Geometry: final body of the model. Coordinates: model frame, mm. Face numbers are marked on the shaded views. A direction names the side the tool comes from. Give positions to 0.01 mm unless a question says otherwise; leave off trailing zeros. Order: outer loops, then holes, each group sorted by start corner. A loop starts at its lowest first (then second) coordinate and runs counter-clockwise, first axis right, second up. Notation, with made-up numbers: M 88,63 L 123,63 A10 cw 123,69 Z; hole C 30.25,10 d11. An arc over 180 degrees is marked long. Write item = value, one per line. Start each with the question number.
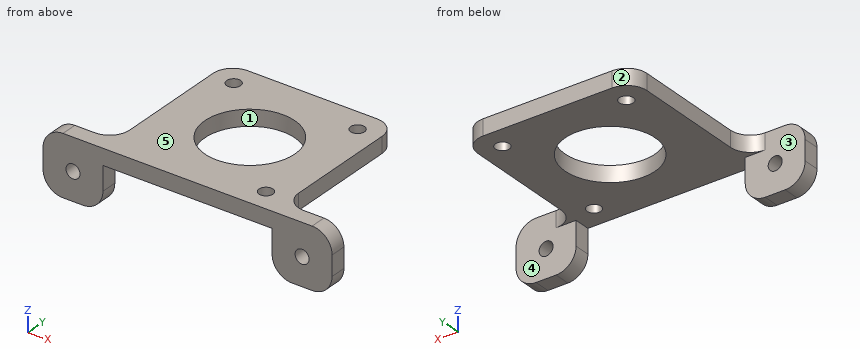
from build123d import *

# Parameters (mm, degrees)
F0_W     = 42.3
F0_H     = 42.2228726387
F0_R     = 1.75
F0_R_2   = 11.25
F1_DEPTH = 4
F2_W     = 15
F2_H     = 4
F3_DEPTH = 15
F4_R     = 5
F5_R     = 1.75
F6_DEPTH = 4


with BuildPart() as f1:
    # F0 (on Top) → F1 (new body)
    with BuildSketch(Plane.XY):
        with Locations((0, 0.0385636806)):
            Rectangle(F0_W, F0_H)
        with Locations((15.495, -15.495)):
            Circle(F0_R, mode=Mode.SUBTRACT)
        Circle(F0_R_2, mode=Mode.SUBTRACT)
        with Locations((-15.495, 15.495)):
            Circle(F0_R, mode=Mode.SUBTRACT)
        with Locations((15.495, 15.495)):
            Circle(F0_R, mode=Mode.SUBTRACT)
    extrude(amount=F1_DEPTH)

    # F2 (on face) → F3 (join)
    with BuildSketch(Plane.XY.offset(4)):
        with Locations((-28.65, -19.0728726387)):
            Rectangle(F2_W, F2_H)
        with Locations((28.65, -19.0728726387)):
            Rectangle(F2_W, F2_H)
    extrude(amount=-F3_DEPTH)

    # F4
    f4_edges = [f1.edges().sort_by_distance(p)[0] for p in [
        (21.15, 21.15, 2),
        (-21.15, 21.15, 2),
        (-21.15, -17.072873, 2),
        (21.15, -17.072873, 2),
        (36.15, -19.072873, 4),
        (-36.15, -19.072873, 4),
        (36.15, -19.072873, -11),
        (21.15, -19.072873, -11),
        (-21.15, -19.072873, -11),
        (-36.15, -19.072873, -11),
    ]]
    fillet(f4_edges, radius=F4_R)

    # F5 (on face) → F6 (cut, through all)
    with BuildSketch(Plane.XZ.offset(21.0728726387)):
        with Locations((-28.65, -4)):
            Circle(F5_R)
        with Locations((28.65, -4)):
            Circle(F5_R)
    extrude(amount=-F6_DEPTH, mode=Mode.SUBTRACT)


solid = f1.part
1) Ray query, L1, parallel to Z at x = 28.65, y = -17.95; L2, parallel to Y at x = -28, z = 1.75; L3, parallel to X at y = 12.5, z = 1.25. Return the intervals inside material, ascending.
2) Draft query along X for the marked faces 1, 2 and 3. Return one class per face: pulls with the +X half, pulls with the -X half, needs draft (parallel to the pull), parting line crosses it, or undercut.
3) Cut plane A-A (y = 0). Return loops of the section in (x, z).
4) Access query for the marked faces 4 and 5. Directions: +Z, -Z, +X, -X, +Y, -Y. A direction counts if a zero-diameter tool reaches every point of the face in a straight line with its end or side. Return the directions, or none.
5) Cut plane D-D (z = 1.25). Return loops of the section in (x, y) (3 decimals), plus the area to 3 significant figures.
6) Pin query (flat end, axial travel): pin 1 Ø5.5 at (x, z) = (-28.65, -4) entering from +Y; pin 2 Ø2 at (x, y) = (-13, -10) entering from -Z; pin 3 Ø1.2 at (y, z) = (3, 1.5) entering from +X. Return the tip coordinate at first contact, or that it passes through.
7) Cut plane B-B (x = 0). Return loops of the section in (y, z).
8) Cut plane C-C (z = -4). Return loops of the section in (x, y).
Reply:
q1.L1 = -11 to -5.75, -2.25 to 4
q1.L2 = -21.07 to -17.07
q1.L3 = -21.15 to 21.15
q2.face_1 = undercut
q2.face_2 = pulls with the -X half
q2.face_3 = needs draft
q3.outline = M -21.15,0 L -11.25,0 L -11.25,4 L -21.15,4 Z; M 11.25,0 L 21.15,0 L 21.15,4 L 11.25,4 Z
q4.face_4 = -Z, +X, +Y
q4.face_5 = +Z, +X, -X, +Y, -Y
q5.outline = M -35.615,-21.073 L 35.615,-21.073 L 35.615,-17.073 L 26.15,-17.073 A5 cw 21.15,-12.073 L 21.15,16.15 A5 ccw 16.15,21.15 L -16.15,21.15 A5 ccw -21.15,16.15 L -21.15,-12.073 A5 cw -26.15,-17.073 L -35.615,-17.073 Z; hole C -15.495,15.495 d3.5; hole C 0,0 d22.5; hole C 15.495,-15.495 d3.5; hole C 15.495,15.495 d3.5
q5.area = 1,480 mm²
q6.pin_1 = -17.07
q6.pin_2 = 0
q6.pin_3 = 21.15
q7.outline = M -21.07,0 L -11.25,0 L -11.25,4 L -21.07,4 Z; M 11.25,0 L 21.15,0 L 21.15,4 L 11.25,4 Z
q8.outline = M -36.15,-21.07 L -30.4,-21.07 L -30.4,-17.07 L -36.15,-17.07 Z; M -26.9,-21.07 L -21.15,-21.07 L -21.15,-17.07 L -26.9,-17.07 Z; M 21.15,-21.07 L 26.9,-21.07 L 26.9,-17.07 L 21.15,-17.07 Z; M 30.4,-21.07 L 36.15,-21.07 L 36.15,-17.07 L 30.4,-17.07 Z
